```python
from build123d import *

# Parameters (mm, degrees)
F0_W     = 66.802
F0_H     = 122.936
F1_DEPTH = 7.112
F2_T     = -2.54
F3_R     = 5.08


with BuildPart() as f1:
    # F0 (on Front) → F1 (new body)
    with BuildSketch(Plane.XZ):
        Rectangle(F0_W, F0_H)
    extrude(amount=F1_DEPTH)

    # F2
    f2_openings = [f1.faces().sort_by_distance(p)[0] for p in [
        (0, -7.112, 0),
    ]]
    offset(amount=F2_T, openings=f2_openings)

    # F3
    f3_edges = [f1.edges().sort_by_distance(p)[0] for p in [
        (33.401, -3.556, 61.468),
        (33.401, -3.556, -61.468),
        (-33.401, -3.556, -61.468),
        (-33.401, -3.556, 61.468),
        (-33.401, 0, 0),
        (0, 0, 61.468),
        (33.401, 0, 0),
        (0, 0, -61.468),
    ]]
    fillet(f3_edges, radius=F3_R)


solid = f1.part
```
Build history of the part. All positions in model axes, mm. A direction names the side the tool comes from. Round coordinates to 2 decimals unless told otherwise and drop trailing zeros. Write each loop counter-clockwise with the first axis right and the second up, starting at its lowest first coordinate (ties: lowest second). Pieces come first, ordered by that corner, then holes. Notation, with made-up numbers: (4.25, -6) -> (53.25, -6) arc R20 cw to (53.25, 0) -> close; hole circle Ø1 at (45, -5.75). An arc over 180 degrees is marked (long way). Put each result on its own line as item: value.
Item 1: Slice it at A-A, the plane x = -10. Give the cut face in (y, z), plus the area to 3 significant figures.
Here are the results:
outline: (-7.11, -61.47) -> (-5.08, -61.47) arc R5.08 ccw to (0, -56.39) -> (0, 56.39) arc R5.08 ccw to (-5.08, 61.47) -> (-7.11, 61.47) -> (-7.11, 58.93) -> (-2.54, 58.93) -> (-2.54, -58.93) -> (-7.11, -58.93) -> close
area: 324 mm^2
Item 2: Wall check: probe 1 along Z at (x, y) = (-2, -5); probe 2 along X at (y, z) = (-6, 18); probe 3 along Y at (x, z) = (-3.5, 25.5). Give the ranges that are in metal, low to high. Write a range as from..to.
Here are the results:
probe 1: z = -61.47..-58.93, 58.93..61.47
probe 2: x = -33.4..-30.86, 30.86..33.4
probe 3: y = -2.54..0
Item 3: Flat gauge pins, fed straight in: P1, Ø4, axis at x = -15.5, z = -23.5, coming from the -Y side; P2, Ø3, axis at y = -2.5, z = -44, coming from the -X side; P3, Ø3, axis at x = -22, y = -3, coming from the +Z side. Where does each tip first touch, or does it go through?
Here are the results:
P1: stops at y = -2.54
P2: stops at x = -33.28
P3: stops at z = 61.43
Item 4: Two-plate mould, pull along X, no slides. Class faces 1 (the face through (-31.952, -1.528, 0.789)), 2 (the face through (0.4, -1.53, 60.02)), 3 (the face through (31.952, -1.528, 0.789)), 4 (the face through (0, -5, -58.928)): pulls with the +X half, pulls with the -X half, needs draft (parallel to the pull), parting line crosses it, or undercut.
Here are the results:
face 1: pulls with the -X half
face 2: needs draft
face 3: pulls with the +X half
face 4: undercut
Item 5: Slice it at B-B, the plane z = -41. Give the cut face in (x, y), plus the area to 3 significant figures.
Here are the results:
outline: (-33.4, -7.11) -> (-30.86, -7.11) -> (-30.86, -2.54) -> (30.86, -2.54) -> (30.86, -7.11) -> (33.4, -7.11) -> (33.4, -5.08) arc R5.08 ccw to (28.32, 0) -> (-28.32, 0) arc R5.08 ccw to (-33.4, -5.08) -> close
area: 182 mm^2
Item 6: Tool access for faces 5 (the face through (30.861, -5, -1)), 6 (the face through (-31.95, -6.11, 59.94)): list every direction of +Z, -Z, +X, -X, +Y, -Y with a clear straight run to the whole face (end or side of a thin tool).
Here are the results:
face 5: -Y
face 6: +Z, -X, +Y, -Y
